Autodesk Fusion 360 part; units mm, degrees
sketch "Sketch1" plane through (0, 0, 0) normal (0, 0, 1) x (1, 0, 0)
  circle A0 centre (0, 0) radius 6.2
  circle A1 centre (0, 0) radius 4
  circle A2 centre (1, 0) radius 2.5
  line L0 (9.5, 0) -> (4.75, 8.2272)
  line L1 (4.75, 8.2272) -> (-4.75, 8.2272)
  line L2 (-4.75, 8.2272) -> (-9.5, 0)
  line L3 (-9.5, 0) -> (-4.75, -8.2272)
  line L4 (-4.75, -8.2272) -> (4.75, -8.2272)
  line L5 (4.75, -8.2272) -> (9.5, 0)
  line L6 (0, 0) -> (1, 0) construction
  circle A3 centre (11.7511, 0) radius 3
  line L7 (9.5, 0) -> (11.7511, 0) construction
  line L8 (8.9226, 1) -> (8.9226, -1) construction
  dimension "d1" = 16.4545
  dimension "d2" = 12.4
  dimension "d3" = 8
  dimension "d4" = 5
  dimension "d5" = 1
  dimension "d6" = 6
  dimension "d7" = 2
extrude "Extrude1" add sketch "Sketch1" along normal blind 8 contours A1
extrude "Extrude2" add sketch "Sketch1" along normal blind 3.5 contours A0 | L0 L1 L2 L3 L4 L5 A3
extrude "Extrude3" add sketch "Sketch1" along normal blind 0.5 from surface at 3.5 contours A0
fillet "Fillet1" radius 0.5 5 edges at (4.75, -8.2272, 1.75) (-4.75, -8.2272, 1.75) (-9.5, 0, 1.75) (-4.75, 8.2272, 1.75) (4.75, 8.2272, 1.75)
fillet "Fillet2" radius 0.5 2 edges at (8.9226, 1, 1.75) (8.9226, -1, 1.75)
sketch "Sketch2" plane through (0, 0, 0) normal (0, 0, 1) x (1, 0, 0)
  circle A0 centre (1, 0) radius 2.5
  arc A1 (8.8128, -1.1903) -> (8.8614, -0.806) centre (8.3798, -0.9403) ccw
  line L0 (8.8128, -1.1903) -> (4.8943, -7.9772)
  arc A2 (4.4613, -8.2272) -> (4.8943, -7.9772) centre (4.4613, -7.7272) ccw
  line L1 (4.4613, -8.2272) -> (-4.4613, -8.2272)
  arc A3 (-4.8943, -7.9772) -> (-4.4613, -8.2272) centre (-4.4613, -7.7272) ccw
  line L2 (-4.8943, -7.9772) -> (-9.3557, -0.25)
  arc A4 (-9.3557, 0.25) -> (-9.3557, -0.25) centre (-8.9226, 0) ccw
  line L3 (-9.3557, 0.25) -> (-4.8943, 7.9772)
  arc A5 (-4.4613, 8.2272) -> (-4.8943, 7.9772) centre (-4.4613, 7.7272) ccw
  line L4 (-4.4613, 8.2272) -> (4.4613, 8.2272)
  arc A6 (4.8943, 7.9772) -> (4.4613, 8.2272) centre (4.4613, 7.7272) ccw
  line L5 (4.8943, 7.9772) -> (8.8128, 1.1903)
  arc A7 (8.8614, 0.806) -> (8.8128, 1.1903) centre (8.3798, 0.9403) ccw
  arc A8 (8.8614, 0.806) -> (8.8614, -0.806) centre (11.7511, 0) ccw
  circle A9 centre (0, 0) radius 4
  circle A10 centre (0, 0) radius 6.2
Verification items for the finished model (mm, model axes). A direction names the side the tool comes from. Round coordinates to 2 decimals unless told otherwise and drop trailing zeros. Loops run counter-clockwise (first coordinate to the right, second up) from the corner with the lowest first, then second, coordinate; pieces in that order, holes last. Notation, with made-up numbers: (77.5, 54) - (95.5, 54) arc R14 ccw to (95.5, 70) - close; hole circle Ø7 at (66.5, 17). An arc over 180 degrees is marked (long way). Write item = value, one per line.
Q1. Sectioned sample at B-B on z = 2. Record the boundary of the cut face in (x, y), plus the area to 3 significant figures.
Here are the results:
outline = (-9.36, -0.25) - (-4.89, -7.98) arc R0.5 ccw to (-4.46, -8.23) - (4.46, -8.23) arc R0.5 ccw to (4.89, -7.98) - (8.81, -1.19) arc R0.5 ccw to (8.86, -0.81) arc R3 cw to (8.86, 0.81) arc R0.5 ccw to (8.81, 1.19) - (4.89, 7.98) arc R0.5 ccw to (4.46, 8.23) - (-4.46, 8.23) arc R0.5 ccw to (-4.89, 7.98) - (-9.36, 0.25) arc R0.5 ccw to start; hole circle Ø5 at (1, 0)
area = 214 mm^2
Q2. Depth check by flat-ended pin: pin 1 (1.5 mm diameter, centred on y = -1, z = 5.5, fed in from +X); pin 2 (2 mm diameter, centred on x = -6.5, z = 2.5, fed in from +Y); pin 3 (1 mm diameter, centred on x = 6.5, z = 6, fed in from +Y). Enter the tip coordinate at first touch or a pass-through.
Here are the results:
pin_1 = 3.99
pin_2 = 6.93
pin_3 = through
Q3. Sectioned sample at C-C on x = 1. Record the boundary of the cut face in (y, z).
Here are the results:
outline = (-8.23, 0) - (-2.5, 0) - (-2.5, 8) - (-3.87, 8) - (-3.87, 4) - (-6.12, 4) - (-6.12, 3.5) - (-8.23, 3.5) - close; (2.5, 0) - (8.23, 0) - (8.23, 3.5) - (6.12, 3.5) - (6.12, 4) - (3.87, 4) - (3.87, 8) - (2.5, 8) - close
Q4. Material ranges on L1, parallel to Y at x = 1, z = 2.75; L2, parallel to Z at x = -3.25, y = -5.75; L3, parallel to Z at x = 2.5, y = -3.5, recorded low to high.
Here are the results:
L1 = -8.23 to -2.5, 2.5 to 8.23
L2 = 0 to 3.5
L3 = 0 to 4
Q5. Sectioned sample at D-D on y = -2.75. Record the boundary of the cut face in (x, z), plus the area to 3 significant figures.
Here are the results:
outline = (-7.91, 0) - (7.91, 0) - (7.91, 3.5) - (5.56, 3.5) - (5.56, 4) - (2.9, 4) - (2.9, 8) - (-2.9, 8) - (-2.9, 4) - (-5.56, 4) - (-5.56, 3.5) - (-7.91, 3.5) - close
area = 84.2 mm^2
Q6. Mould release check, pull along X, two halves, no side actions. Record for faces 1 (the flat face through (0, 8.227, 2)), 2 (the flat face through (-7.094, 4.168, 1.726)), 3 (the cylindrical face through (3.31, 0.96, 3.94)): +X half, -X half, draft (parallel to the pull), parting line (faces both ways), or undercut.
Here are the results:
face_1 = draft
face_2 = -X half
face_3 = undercut
Q7. Tool access check on faces 4 (the flat face through (-7.156, -4.06, 1.726)), 5 (the cylindrical face through (-0.867, 3.905, 5.972)). Record the directions out of +Z, -Z, +X, -X, +Y, -Y that give a thin tool (end or side, any length) a straight path to the whole face; none if there is none.
Here are the results:
face_4 = +Z, -Z, -X, -Y
face_5 = +Z
Q8. Sectioned sample at A-A on y = 0. Record the boundary of the cut face in (x, z), plus the area to 3 significant figures.
Here are the results:
outline = (-9.42, 0) - (-1.5, 0) - (-1.5, 8) - (-4, 8) - (-4, 4) - (-6.2, 4) - (-6.2, 3.5) - (-9.42, 3.5) - close; (3.5, 0) - (8.75, 0) - (8.75, 3.5) - (6.2, 3.5) - (6.2, 4) - (4, 4) - (4, 8) - (3.5, 8) - close
area = 61.8 mm^2
